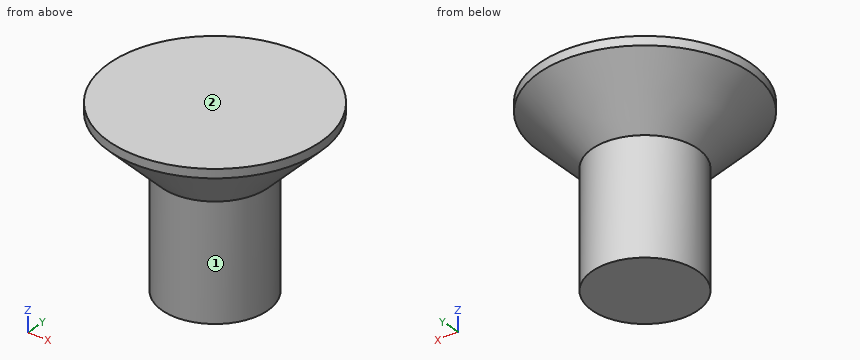
Autodesk Inventor part; units mm, degrees
ref_plane "YZ Plane" through (0, 0, 0) normal (1, 0, 0) x (0, 1, 0)
ref_plane "XZ Plane" through (0, 0, 0) normal (0, 1, 0) x (-1, 0, 0)
ref_plane "XY Plane" through (0, 0, 0) normal (0, 0, 1) x (1, 0, 0)
sketch "スケッチ1" plane through (0, 0, 0) normal (0, 0, 1) x (1, 0, 0)
  circle A0 centre (0, 0) radius 1.5
  dimension "d0" = 3
extrude "押し出し1" add sketch "スケッチ1" along normal blind 6
sketch "スケッチ2" plane through (0, 0, 6) normal (0, 0, 1) x (1, 0, 0)
  circle A0 centre (0, 0) radius 1.5
  circle A1 centre (0, 0) radius 3
  dimension "d3" = 6
extrude "押し出し2" add sketch "スケッチ2" along normal blind 1.75 contours A0 | A1
thread "ねじ1"
chamfer "面取り1" distance 1.5 angle 45 1 edges at (-3, 0, 6)
sketch "スケッチ4" plane through (0, 0, 0) normal (0, 0, -1) x (-1, 0, 0)
  circle A0 centre (0, 0) radius 1.5
extrude "押し出し4" cut sketch "スケッチ4" against normal blind 2
sketch "スケッチ5" plane through (0, 0, 2) normal (0, 0, -1) x (-1, 0, 0)
  circle A0 centre (0, 0) radius 1.5
extrude "押し出し5" cut sketch "スケッチ5" against normal blind 0.75
properties part number "SB　5mm皿ネジ" material "Steel, Mild"
Could you check a few things on this model? Use its own coordinates, in mm. Face numbers are marked on the shaded views. A direction names the side the tool comes from. Give positions to 0.01 mm unless a question says otherwise; leave off trailing zeros. Order: outer loops, then holes, each group sorted by start corner. A loop starts at its lowest first (then second) coordinate and runs counter-clockwise, first axis right, second up.
1. I need wall thicknesses on L1, parallel to Z at x = -2.5, y = 1.25; L2, parallel to Z at x = 0.95, y = 1.45; L3, parallel to X at y = 0.3, z = 6.35. Which ranges of each line are inside material? Lowest first, please.
Answers below:
L1: z = 7.29 to 7.75
L2: z = 6.23 to 7.75
L3: x = -1.83 to 1.83
2. Suppose I cut it at C-C (z = 3.15). Write out the boundary of the cut face in (x, y), plus the area to 3 significant figures.
Answers below:
outline: circle Ø3 at (0, 0)
area: 7.07 mm2
3. For pin 1 (2 mm diameter, centred on x = 1, z = 6.5, fed in from +Y); pin 2 (1.5 mm diameter, centred on y = 2, z = 4, fed in from -X), each with a flat end and sliding along its axis, tell me the tip position at first contact or that it passes through.
Answers below:
pin 1: stops at y = 2.87
pin 2: stops at x = -0.83
4. Which directions (+Z, -Z, +X, -X, +Y, -Y) give clear straight access to the entire face, cutting with the end or side of a thin tool? Please do the marked faces 1 and 2.
Answers below:
face 1: -Z
face 2: +Z, +X, -X, +Y, -Y
5. Suppose I cut it at D-D (z = 6.4). Write out the boundary of the cut face in (x, y).
Answers below:
outline: circle Ø3.8 at (0, 0)
